Part model, mm, in its own coordinate system. Face numbers are marked on the shaded views. Round coordinates to 2 decimals unless told otherwise and drop trailing zeros. Loops run counter-clockwise (first coordinate to the right, second up) from the corner with the lowest first, then second, coordinate; pieces in that order, holes last. Notation, with made-up numbers: (-34.5, 17.5) -> (-26.5, 17.5) arc R24 cw to (-26.5, 31.5) -> close; hole circle Ø9 at (-2.5, -37.5). An arc over 180 degrees is marked (long way). Use a Markdown table: item, result. Add a question column.
Item 1: Cut at C-C, the plane z = 29. List the corners of the cut face in (x, y), plus the area to 4 significant figures.
Item 2: Probe line 1 (Y direction, x = 24, z = -21.5). List the from-to ranges inside material, lowest first. Write a range as [from, to].
Item 3: Two-plate mould, pull along Y, no slides. Class the marked faces 1 and 2: pulls with the +Y half, pulls with the -Y half, needs draft (parallel to the pull), parting line crosses it, or undercut.
Item 4: Flat gauge pins, fed straight in: pin 1 (10 mm diameter, centred on x = -46, z = 36.5, fed in from -Y); pin 2 (1.4 mm diameter, centred on x = -61.5, y = -0.5, fed in from -Z); pin 3 (0.6 mm diameter, centred on x = -62, y = -1, fed in from +Z) (3 decimals). Where does each tip first touch, or does it go through?
Item 5: Cut at B-B, the plane x = -47. List the corners of the cut face in (y, z), plus the area to 3 significant figures.
Item 6: Cut at A-A, the plane z = 13.8. List the corners of the cut face in (x, y).
```python
from build123d import *

# Parameters (mm, degrees)
SKETCH2_W           = 132.6
SKETCH2_H           = 95.6
BOSS_EXTRUDE1_DEPTH = 2.5
CHAMFER1_SIZE       = 2
BOSS_EXTRUDE2_DEPTH = 1.3


with BuildPart() as part:
    # Sketch2 → Boss-Extrude1 (new body)
    with BuildSketch(Plane(origin=(0, 0, 0), x_dir=(1, 0, 0), z_dir=(0, 1, 0))):
        Rectangle(SKETCH2_W, SKETCH2_H)
    extrude(amount=BOSS_EXTRUDE1_DEPTH)

    # Chamfer1
    chamfer1_edges = [part.edges().sort_by_distance(p)[0] for p in [
        (66.3, 1.25, 47.8),
        (-66.3, 1.25, 47.8),
        (-66.3, 1.25, -47.8),
        (66.3, 1.25, -47.8),
    ]]
    chamfer(chamfer1_edges, length=CHAMFER1_SIZE)

    # Sketch3 → Boss-Extrude2 (add)
    with BuildSketch(Plane.XZ):
        with BuildLine():
            Line((-58.425, 18.925), (-66.3, 18.925))
            Line((-66.3, 18.925), (-66.3, 8.675))
            Line((-66.3, 8.675), (-58.425, 8.675))
            ThreePointArc((-58.425, 8.675), (-53.3, 13.8), (-58.425, 18.925))
        make_face()
    extrude(amount=BOSS_EXTRUDE2_DEPTH)


solid = part.part
```
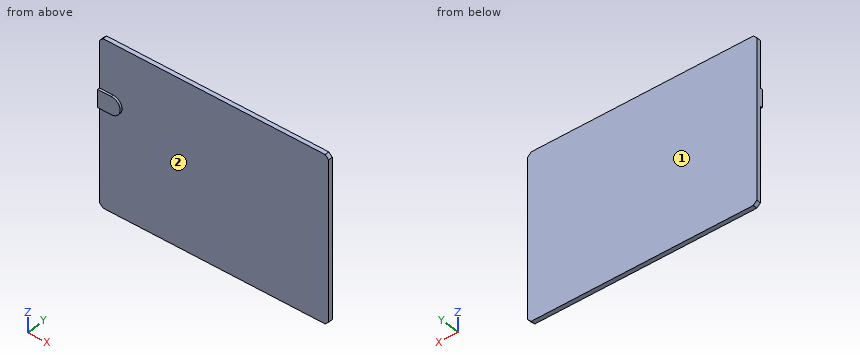
A:
| question | item | result |
|---|---|---|
| 1 | outline | (-66.3, 0) -> (66.3, 0) -> (66.3, 2.5) -> (-66.3, 2.5) -> close |
| 1 | area | 331.5 mm^2 |
| 2 | line 1 | y = [0, 2.5] |
| 3 | face 1 | pulls with the +Y half |
| 3 | face 2 | pulls with the -Y half |
| 4 | pin 1 | stops at y = 0 |
| 4 | pin 2 | stops at z = -47.8 |
| 4 | pin 3 | stops at z = 18.925 |
| 5 | outline | (0, -47.8) -> (2.5, -47.8) -> (2.5, 47.8) -> (0, 47.8) -> close |
| 5 | area | 239 mm^2 |
| 6 | outline | (-66.3, -1.3) -> (-53.3, -1.3) -> (-53.3, 0) -> (66.3, 0) -> (66.3, 2.5) -> (-66.3, 2.5) -> close |
